Part model, mm, in its own coordinate system. A direction names the side the tool comes from. Round coordinates to 2 decimals unless told otherwise and drop trailing zeros. Loops run counter-clockwise (first coordinate to the right, second up) from the corner with the lowest first, then second, coordinate; pieces in that order, holes last.
1) Drop flat-ended pins along their axis: P1, Ø11.5, axis at x = 0, z = 250, coming from the -Y side; P2, Ø15, axis at x = -4.5, z = 248.5, coming from the -Y side; P3, Ø7.5, axis at x = -6, z = 181, coming from the +Y side; P4, Ø8, axis at x = 4, y = 2, coming from the -Z side. Give the stop position or say it passes through.
2) Band-saw the part on B-B, the plane z = 102.5. Write the cut outline in (x, y).
3) 3-axis set-ups, long thin cutter, end or side, ignore diameter. For faces 1 (the flat face through (2, -10.5, 0)), 2 (the cylindrical face through (-1.08, -8.98, 4.88)), 3 (the flat face through (-4, 7.5, -4)): which of +Z, -Z, +X, -X, +Y, -Y reach the whole face in a straight line?
4) Band-saw the part on A-A, the plane z = 250. Write the cut outline in (x, y), then the cut area to 3 significant figures.
5) Mould opens along Z. For faces 4 (the cylindrical face through (-6, -6, 0)), 5 (the cylindrical face through (-2.059, -1.049, 240.726)), 6 (the flat face through (0, -4.5, 128)), 7 (the flat face through (-2.2, 2.5, 241.6)) say: +Z half, -Z half, draft (parallel to the pull), parting line (faces both ways), or undercut.
6) Probe line 1 (Z direction, x = 0, y = 3.5); line 2 (Z direction, x = 0, y = -0.5); line 3 (Y direction, x = 3.5, z = 92). List the from-to ranges inside material, lowest first.
from build123d import *

# Parameters (mm, degrees)
SKETCH_1_R           = 5
EXTRUDE_1_DEPTH      = 10.5
EXTRUDE_1_DEPTH_BACK = 10.5
EXTRUDE_3_DEPTH      = 4.5
EXTRUDE_3_DEPTH_BACK = 4.5
SKETCH_7_R           = 6
EXTRUDE_4_DEPTH      = 3
SKETCH_8_R           = 6
EXTRUDE_5_DEPTH      = 3
SKETCH_9_R           = 9.5
CUT_EXTRUDE_1_DEPTH  = 7
SKETCH_10_R          = 8.5
CUT_EXTRUDE_2_DEPTH  = 9
HOLE_WIZARD_M4_1_D   = 3.3


with BuildPart() as part:
    # Sketch 1 → Extrude 1 (new body, two sides)
    with BuildSketch(Plane(origin=(0, 0, 0), x_dir=(1, 0, 0), z_dir=(0, 1, 0))) as extrude_1_sk:
        Circle(SKETCH_1_R)
    extrude(amount=EXTRUDE_1_DEPTH)
    extrude(extrude_1_sk.sketch, amount=-EXTRUDE_1_DEPTH_BACK)

    # Sketch 6 → Extrude 3 (add, two sides)
    with BuildSketch(Plane(origin=(0, 0, 0), x_dir=(1, 0, 0), z_dir=(0, 1, 0))) as extrude_3_sk:
        with BuildLine():
            Line((-12.5, 0), (-12.5, -260))
            ThreePointArc((-12.5, -260), (0, -272.5), (12.5, -260))
            Line((12.5, -260), (12.5, 0))
            ThreePointArc((12.5, 0), (0, 12.5), (-12.5, 0))
        make_face()
    extrude(amount=EXTRUDE_3_DEPTH)
    extrude(extrude_3_sk.sketch, amount=-EXTRUDE_3_DEPTH_BACK)

    # Sketch 7 → Extrude 4 (add)
    with BuildSketch(Plane.XZ.offset(4.5)):
        Circle(SKETCH_7_R)
    extrude(amount=EXTRUDE_4_DEPTH)

    # Sketch 8 → Extrude 5 (add)
    with BuildSketch(Plane(origin=(0, 4.5, 0), x_dir=(1, 0, 0), z_dir=(0, 1, 0))):
        Circle(SKETCH_8_R)
    extrude(amount=EXTRUDE_5_DEPTH)

    # Sketch 9 → Cut-Extrude 1 (cut)
    with BuildSketch(Plane.XZ.offset(4.5)):
        with Locations((0, 250)):
            Circle(SKETCH_9_R)
    extrude(amount=-CUT_EXTRUDE_1_DEPTH, mode=Mode.SUBTRACT)

    # Sketch 10 → Cut-Extrude 2 (cut, through all)
    with BuildSketch(Plane.XZ.offset(-2.5)):
        with Locations((0, 250)):
            Circle(SKETCH_10_R)
    extrude(amount=-CUT_EXTRUDE_2_DEPTH, mode=Mode.SUBTRACT)

    # Hole Wizard M4 _ _ _ _1 (through all)
    with Locations(Plane(origin=(0, -10.5, 0), x_dir=(-1, 0, 0), z_dir=(0, -1, 0))):
        with Locations((0, 0)):
            Hole(HOLE_WIZARD_M4_1_D / 2)


solid = part.part
Reported:
1. P1: passes through
1. P2: stops at y = -4.5
1. P3: stops at y = 4.5
1. P4: stops at z = -12.5
2. outline: (-12.5, -4.5) - (12.5, -4.5) - (12.5, 4.5) - (-12.5, 4.5) - close
3. face 1: +Z, -Z, +X, -X, -Y
3. face 2: -Y
3. face 3: +Y
4. outline: (-12.5, -4.5) - (-9.5, -4.5) - (-9.5, 2.5) - (-8.5, 2.5) - (-8.5, 4.5) - (-12.5, 4.5) - close; (8.5, 2.5) - (9.5, 2.5) - (9.5, -4.5) - (12.5, -4.5) - (12.5, 4.5) - (8.5, 4.5) - close
4. area: 58.0 mm2
5. face 4: parting line
5. face 5: undercut
5. face 6: draft
5. face 7: undercut
6. line 1: z = -12.5 to -1.65, 1.65 to 241.5, 258.5 to 272.5
6. line 2: z = -12.5 to -1.65, 1.65 to 240.5, 259.5 to 272.5
6. line 3: y = -4.5 to 4.5
